```python
from build123d import *

# Parameters (mm, degrees)
OUTTER_R          = 11.557
BODY_DEPTH        = 1.524
SCREW_HOLES_COUNT = 4


with BuildPart() as part:
    # outter → Body (new body)
    with BuildSketch(Plane(origin=(0, 0, 0), x_dir=(1, 0, 0), z_dir=(0, 1, 0))):
        with Locations(Location((0, 0, 0), (0, 0, 270))):
            Circle(OUTTER_R)
    extrude(amount=-BODY_DEPTH)

    # Sketch12 → 0 Clearance Hole (revolve, cut)
    with BuildSketch(Plane(origin=(0, 0, -10.541), x_dir=(0, 0, 1), z_dir=(1, 0, 0))):
        Polygon((0, 0), (0, 2.05816509), (0.889, 1.524), (0.889, 0), align=None)
    f_0_clearance_hole = revolve(axis=Axis((0, 6.35, -10.541), (0, -1, 0)), mode=Mode.SUBTRACT)

    # Screw Holes: 0 Clearance Hole ×4 about axis
    screw_holes_axis = Axis((0, 0, 0), (0, 1, 0))
    for i in range(1, SCREW_HOLES_COUNT):
        add(f_0_clearance_hole.rotate(screw_holes_axis, i * 360 / SCREW_HOLES_COUNT), mode=Mode.SUBTRACT)


solid = part.part
```
Part model, mm, in its own coordinate system. Give positions to 0.01 mm unless a question says otherwise; leave off trailing zeros. Write each loop counter-clockwise with the first axis right and the second up, starting at its lowest first coordinate (ties: lowest second). Pieces come first, ordered by that corner, then holes. Notation, with made-up numbers: (27, 54.5) -> (76, 54.5) arc R26 cw to (76, 85.5) -> close; hole circle Ø10 at (79, 6). An arc over 180 degrees is marked (long way). Put each result on its own line as item: value. Start each with the question number.
Item 1: Cut at A-A (x = 0). List the corners of the cut face in (y, z).
Item 2: Cut at B-B (y = -0.5). List the corners of the cut face in (x, z).
Item 3: Pin check, flat tip, straight feed: pin 1 Ø2.5 at (x, z) = (10.541, 0) entering from -Y. Stop position of the tip, or through.
Item 4: Wall check: L1, parallel to X at y = -0.35, z = 0.5; L2, parallel to Z at x = 0.75, y = -0.35; L3, parallel to X at y = -0.45, z = 10.5. Give the ranges that are in metal, low to high. Write a range as [from, to].
Item 5: Cut at C-C (z = 4.5). List the corners of the cut face in (x, y).
Item 6: Cut at D-D (x = 8.25). List the corners of the cut face in (y, z), then the cut area to 3 significant figures.
Item 7: Pull direction Z, two halves, no side cores. Call faces 1 (the face through (-0.541, -0.751, 11.246)), 2 (the face through (0, -1.524, 0)), 3 (the face through (9.745, -0.751, 6.213)): pulls with the +Z half, pulls with the -Z half, needs draft (parallel to the pull), parting line crosses it, or undercut.
Answer list:
1. outline: (-1.52, -11.56) -> (0, -11.56) -> (0, -11.43) -> (-1.52, -11.43) -> close; (-1.52, -9.65) -> (0, -9.65) -> (0, 9.65) -> (-1.52, 9.65) -> close; (-1.52, 11.43) -> (0, 11.43) -> (0, 11.56) -> (-1.52, 11.56) -> close
2. outline: circle Ø23.11 at (0, 0); hole circle Ø1.78 at (-10.54, 0); hole circle Ø1.78 at (0, -10.54); hole circle Ø1.78 at (0, 10.54); hole circle Ø1.78 at (10.54, 0)
3. pin 1: stops at y = -1.52
4. L1: x = [-11.55, -11.28], [-9.81, 9.81], [11.28, 11.55]
4. L2: z = [-11.53, -11.02], [-10.06, 10.06], [11.02, 11.53]
4. L3: x = [-4.83, -0.89], [0.89, 4.83]
5. outline: (-10.64, -1.52) -> (10.64, -1.52) -> (10.64, 0) -> (-10.64, 0) -> close
6. outline: (-1.52, -8.09) -> (0, -8.09) -> (0, 8.09) -> (-1.52, 8.09) -> close
6. area: 24.7 mm2
7. face 1: undercut
7. face 2: needs draft
7. face 3: parting line crosses it
